CAD build for the part. Positions are in the model's coordinates, mm. A direction names the side the tool comes from. Round coordinates to 2 decimals unless told otherwise and drop trailing zeros. Order: outer loops, then holes, each group sorted by start corner. A loop starts at its lowest first (then second) coordinate and runs counter-clockwise, first axis right, second up. Notation, with made-up numbers: M 29.25,6 L 64.25,6 A19 cw 64.25,13 Z; hole C 8.25,67 d2. An arc over 180 degrees is marked long. Put each result on its own line as item: value.
```python
from build123d import *

# Parameters (mm, degrees)
EXTRUDE_1_DEPTH     = 70
CUT_EXTRUDE_1_REACH = 120.788
SKETCH_2_R          = 1.5


with BuildPart() as part:
    # 草图1 → 凸台-拉伸1 (new body)
    with BuildSketch(Plane.XY):
        Polygon((47.658749939, 6.237878975), (-48.93383269, -19.644025535), (-48.93383269, -16.644025535), (44.658749939, 8.434031398), (44.658749939, 21.237878975), (47.658749939, 21.237878975), (47.658749939, 9.237878975), align=None)
    extrude(amount=EXTRUDE_1_DEPTH)

    # 草图2 → 切除-拉伸1 (cut, up to next)
    with BuildSketch(Plane.ZY.offset(-44.658749939), mode=Mode.PRIVATE) as cut_extrude_1_sk1:
        with Locations(Location((5, 14.835955186, 0), (0, 0, 270))):
            Circle(SKETCH_2_R)
    cut_extrude_1_tool1 = extrude(cut_extrude_1_sk1.sketch, amount=-CUT_EXTRUDE_1_REACH, mode=Mode.PRIVATE) & part.part
    # 草图2 → 切除-拉伸1 (cut, up to next)
    with BuildSketch(Plane.ZY.offset(-44.658749939), mode=Mode.PRIVATE) as cut_extrude_1_sk2:
        with Locations(Location((65, 14.835955186, 0), (0, 0, 270))):
            Circle(SKETCH_2_R)
    cut_extrude_1_tool2 = extrude(cut_extrude_1_sk2.sketch, amount=-CUT_EXTRUDE_1_REACH, mode=Mode.PRIVATE) & part.part
    add(cut_extrude_1_tool1.solids().sort_by_distance((44.65875, 14.835955, 5))[0], mode=Mode.SUBTRACT)
    add(cut_extrude_1_tool2.solids().sort_by_distance((44.65875, 14.835955, 65))[0], mode=Mode.SUBTRACT)


solid = part.part
```
Item 1: Band-saw the part on A-A on z = 5. Give the cut face in (x, y).
Answers below:
outline: M -48.93,-19.64 L 47.66,6.24 L 47.66,13.34 L 44.66,13.34 L 44.66,8.43 L -48.93,-16.64 Z; M 44.66,16.34 L 47.66,16.34 L 47.66,21.24 L 44.66,21.24 Z
Item 2: Pin check, flat tips, straight feed: P1, Ø2.5, axis at y = 14.84, z = 65, coming from the -X side; P2, Ø10, axis at y = 15, z = 25, coming from the -X side; P3, Ø3, axis at y = 6, z = 49.5, coming from the +X side; P4, Ø6, axis at x = -26.5, z = 62, coming from the -Y side. Stop position of each tip, or through.
Answers below:
P1: through
P2: x = 44.66
P3: x = 47.66
P4: y = -14.44
Item 3: Band-saw the part on B-B on z = 20. Give the cut face in (x, y), and give its area (3 significant figures).
Answers below:
outline: M -48.93,-19.64 L 47.66,6.24 L 47.66,21.24 L 44.66,21.24 L 44.66,8.43 L -48.93,-16.64 Z
area: 327 mm²
Item 4: Band-saw the part on D-D on x = 16. Give the cut face in (y, z), and give its area (3 significant figures).
Answers below:
outline: M -2.25,0 L 0.75,0 L 0.75,70 L -2.25,70 Z
area: 210 mm²
Item 5: Band-saw the part on C-C on y = 9.5. Give the cut face in (x, z).
Answers below:
outline: M 44.66,0 L 47.66,0 L 47.66,70 L 44.66,70 Z
Item 6: Tool access for faces 1 (the flat face through (44.659, 15, 35)), 2 (the flat face through (7, -2, 70)): list every direction of +Z, -Z, +X, -X, +Y, -Y with a clear straight run to the whole face (end or side of a thin tool).
Answers below:
face 1: +Z, -Z, -X, +Y
face 2: +Z, +X, -X, +Y, -Y
Item 7: Mould opens along Z. For faces 3 (the flat face through (-2.79, -4.28, 34.51)), 4 (the cylindrical face through (46.138, 15.942, 66.014)), 5 (the cylindrical face through (46.138, 16.335, 5.066)), 6 (the flat face through (7, -2, 0)) say: pulls with the +Z half, pulls with the -Z half, needs draft (parallel to the pull), parting line crosses it, or undercut.
Answers below:
face 3: needs draft
face 4: undercut
face 5: undercut
face 6: pulls with the -Z half
Item 8: Probe line 1 along Y through (x, z) = (45, 65); line 2 along X through (y, z) = (19, 42); line 3 along Y through (x, z) = (42, 9). List the from-to ranges inside material, lowest first. Write a range as [from, to].
Answers below:
line 1: [5.53, 13.34], [16.34, 21.24]
line 2: [44.66, 47.66]
line 3: [4.72, 7.72]
